For this review, take the finished solid that the model builds, in its own axes (mm). Face numbers are marked on the shaded views. Give positions to 0.01 mm unless a question says otherwise; leave off trailing zeros. Order: outer loops, then holes, each group sorted by start corner. A loop starts at its lowest first (then second) coordinate and runs counter-clockwise, first axis right, second up. Notation, with made-up numbers: (-39, 69.5) -> (-15, 69.5) arc R25 ccw to (-15, 106.5) -> close; hole circle Ø2 at (79.5, 54). An arc over 180 degrees is marked (long way). Return JSON: item names as keys, results as strings. Group by question number.
1) Add section D-D (x = 113.5). Give the boundary of the cut face in (y, z).
2) Add section B-B (y = -2). Give the boundary of the cut face in (x, z).
3) Add section C-C (x = -2). Give the boundary of the cut face in (y, z).
4) To check wall thickness, follow line 1 along Y through (x, z) = (52.5, -7.25); line 2 along Z through (x, y) = (31, 1.5); line 3 along Z through (x, y) = (41, 2). State the ranges of each line that lie inside material, in increasing order.
5) Insertion check: P1, Ø2, axis at x = 120, z = -2, coming from the +Y side; P2, Ø3, axis at x = 99, z = 10, coming from the -Y side; P3, Ø1.5, axis at x = -16.5, y = 6.5, coming from the +Z side; P4, Ø3, axis at y = -3, z = -1.5, coming from the -X side. Each pin has a flat end and moves straight along its axis. Give the tip position at first contact, or say it passes through.
6) The part is to be moulded in two halves that separate along Y. For the marked faces 1 and 2, say which applies: released by +Y, released by -Y, zero draft, split by the parting line, or undercut.
7) Add section A-A (z = 0). Give the boundary of the cut face in (x, y).
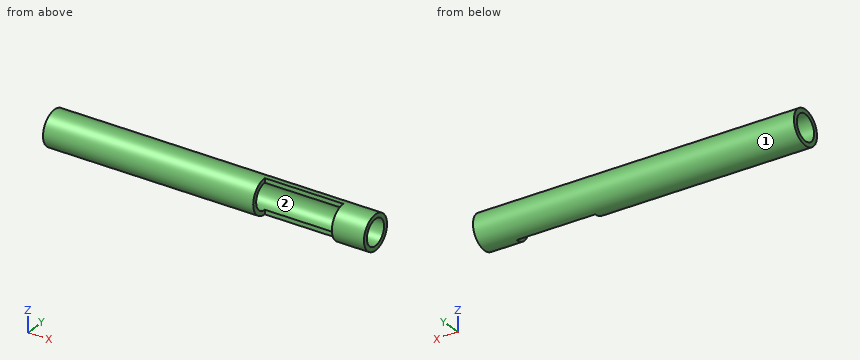
from build123d import *

# Parameters (mm, degrees)
F0_W     = 131
F0_H     = 10.75
F0_W_2   = 49
F0_W_3   = 20
F2_R     = 8
F3_DEPTH = 300
F4_DEPTH = 13


with BuildPart() as f1:
    # F0 (on Top) → F1 (revolve)
    with BuildSketch(Plane.XY):
        with Locations((6.6921378869, -2.8394986279)):
            Rectangle(F0_W, F0_H)
        with Locations((96.6921378869, -2.8394986279)):
            Rectangle(F0_W_2, F0_H)
        with Locations((131.1921378869, -2.8394986279)):
            Rectangle(F0_W_3, F0_H)
    revolve(axis=Axis((41.1921378869, 2.5355013721, 0), (1, 0, 0)))

    # F2 (on face) → F3 (cut)
    with BuildSketch(Plane(origin=(-58.8078621131, 0, 0), x_dir=(0, -1, 0), z_dir=(-1, 0, 0))):
        with Locations((-2.5355013721, 0)):
            Circle(F2_R)
    extrude(amount=-F3_DEPTH, mode=Mode.SUBTRACT)

    # F0 (on Top) → F4 (cut, symmetric)
    with BuildSketch(Plane.XY):
        with Locations((96.6921378869, -2.8394986279)):
            Rectangle(F0_W_2, F0_H)
    extrude(amount=F4_DEPTH, both=True, mode=Mode.SUBTRACT)


solid = f1.part
Evaluation:
{
 "1": {"outline": "(2.54, -10.75) arc R10.75 ccw to (2.54, 10.75) -> (2.54, 8) arc R8 cw to (2.54, -8) -> close"},
 "2": {"outline": "(-58.81, -9.75) -> (72.19, -9.75) -> (72.19, -6.59) -> (-58.81, -6.59) -> close; (-58.81, 6.59) -> (72.19, 6.59) -> (72.19, 9.75) -> (-58.81, 9.75) -> close; (121.19, -9.75) -> (141.19, -9.75) -> (141.19, -6.59) -> (121.19, -6.59) -> close; (121.19, 6.59) -> (141.19, 6.59) -> (141.19, 9.75) -> (121.19, 9.75) -> close"},
 "3": {"outline": "circle Ø21.5 at (2.54, 0); hole circle Ø16 at (2.54, 0)"},
 "4": {"line 1": "-5.4 to -0.85, 5.92 to 10.47", "line 2": "-10.7 to -7.93, 7.93 to 10.7", "line 3": "-10.74 to -7.98, 7.98 to 10.74"},
 "5": {"P1": "y = 13.24", "P2": "y = 2.54", "P3": "z = 10.26", "P4": "through"},
 "6": {"face 1": "split by the parting line", "face 2": "undercut"},
 "7": {"outline": "(-58.81, -8.21) -> (72.19, -8.21) -> (72.19, -5.46) -> (-58.81, -5.46) -> close; (-58.81, 10.54) -> (141.19, 10.54) -> (141.19, 13.29) -> (-58.81, 13.29) -> close; (121.19, -8.21) -> (141.19, -8.21) -> (141.19, -5.46) -> (121.19, -5.46) -> close"}
}
